Study the drawing (mm; zero at the part's minimum x, y, z) and answer. A direction names the side the tool comes from. Coordinates: 2 decimals unless noted, no trailing zeros. Order: outer loops, then holes, each group sorted by start corner. A loop starts at its lowest first (then second) coordinate and runs counter-clockwise, first axis right, second up. Notation, with made-up numbers: (-33, 4.5) -> (13, 4.5) arc R21 ccw to (13, 12.5) -> close; hole circle Ø5 at (36, 3). An arc over 180 degrees is marked (long way). Write each question's results on one line, items separated by ' | '. Start each with the question number.
(1) Given pin 1 (12 mm diameter, centred on x = 495.5, y = 325, fed in from -Z); pin 2 (1 mm diameter, centred on x = 859.5, y = 546, fed in from +Z); pin 3 (12 mm diameter, centred on x = 1276, y = 152.5, fed in from +Z), each flat-ended and moving along its own axis, determine where each tip first touches the part or whether it passes through.
(2) The part is cut by section A-A, the plane z = 350. Give the vertices of the cut face in (x, y).
(3) Straight lines are drawn through the part: L1, parallel to X at y = 411.5, z = 350; L2, parallel to Z at x = 1237, y = 339; L3, parallel to X at y = 163, z = 122.5. For each, find the intervals that lie inside material, in ascending order.
(4) A tool of negligible diameter and unlimited length cuts with its end or side. For the marked faces 1 and 2, from which of +Z, -Z, +X, -X, +Y, -Y can it reach the whole face along a straight path? Write none if from no direction.
(5) The part is cut by section B-B, the plane y = 335. Give the vertices of the cut face in (x, z), then the cut area to 3 significant figures.
(6) The part is cut by section D-D, the plane x = 1420. Give the vertices of the cut face in (y, z).
(7) The part is cut by section C-C, the plane z = 490.5. Give the vertices of the cut face in (x, y), then the cut area to 3 significant figures.
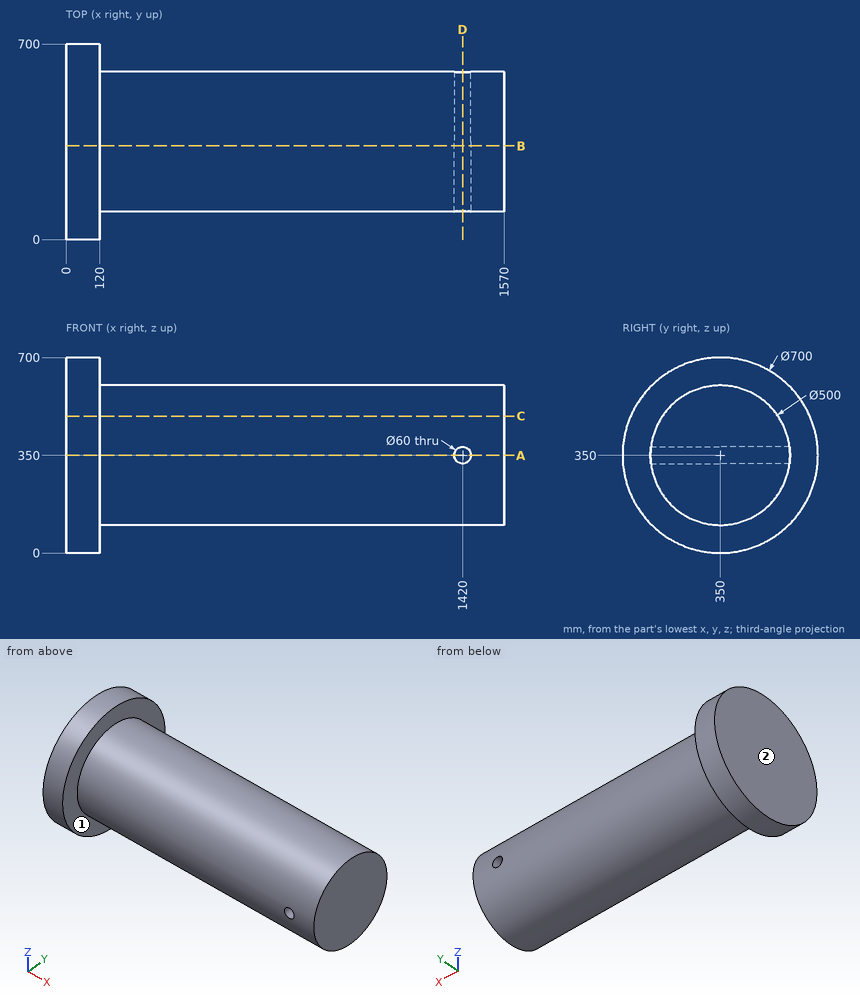
Established:
1) pin 1: stops at z = 100.72 | pin 2: stops at z = 505.82 | pin 3: stops at z = 510.71
2) outline: (0, 0) -> (120, 0) -> (120, 100) -> (1390, 100) -> (1390, 600) -> (120, 600) -> (120, 700) -> (0, 700) -> close; (1450, 100) -> (1570, 100) -> (1570, 600) -> (1450, 600) -> close
3) L1: x = 0 to 1390, 1450 to 1570 | L2: z = 100.24 to 599.76 | L3: x = 0 to 120
4) face 1: +X | face 2: +Z, -Z, -X, +Y, -Y
5) outline: (0, 0.32) -> (120, 0.32) -> (120, 100.45) -> (1570, 100.45) -> (1570, 599.55) -> (120, 599.55) -> (120, 699.68) -> (0, 699.68) -> close; hole circle Ø60 at (1420, 350) | area: 805,000 mm^2
6) outline: (101.81, 320) arc R250 ccw to (598.19, 320) -> close; (101.81, 380) -> (598.19, 380) arc R250 ccw to start
7) outline: (0, 29.44) -> (120, 29.44) -> (120, 143.22) -> (1570, 143.22) -> (1570, 556.78) -> (120, 556.78) -> (120, 670.56) -> (0, 670.56) -> close | area: 677,000 mm^2
